```python
from build123d import *

# Parameters (mm, degrees)
F0_W        = 44.3030558527
F0_H        = 33.7232230231
F0_W_2      = 0.2780174837
F0_H_2      = 4.7262893058
F1_DEPTH    = 46.482
F2_T1_DEPTH = 280.6193273788
F3_R        = 21.4623585695
F4_T1_DEPTH = 270.9255150881
F6_DEPTH    = 40.132


# Not quite as in the source:
# - a fillet or chamfer that OpenCascade refuses, or shapes differently, is made with other operations: its cross-section is extruded or revolved along the edge and cut away or added


with BuildPart() as f1:
    # F0 (on Top) → F1 (new body)
    with BuildSketch(Plane.XY):
        with Locations((0.330619514, -6.2817768194)):
            Rectangle(F0_W, F0_H)
        with Locations((8.0964784138, -9.5091590192)):
            Rectangle(F0_W_2, F0_H_2, mode=Mode.SUBTRACT)
    extrude(amount=F1_DEPTH)

    # F2: fillet of radius 49.6700298323 on 1 edges, made by hand

    # F2_s2 → F2_t1 (cut)
    with BuildSketch(Plane.XZ.offset(-134.02788687)):
        with BuildLine():
            ThreePointArc((-21.8209084123, -2.8972208711), (-9.1217429277, 30.2730527625), (22.4821474403, 46.482))
            Line((22.4821474403, 46.482), (-21.8209084123, 46.482))
            Line((-21.8209084123, 46.482), (-21.8209084123, -2.8972208711))
        make_face()
    extrude(amount=F2_T1_DEPTH, mode=Mode.SUBTRACT)

    # F3
    f3_edges = [f1.edges().sort_by_distance(p)[0] for p in [
        (22.482147, -23.143388, 23.241),
    ]]
    fillet(f3_edges, radius=F3_R)

    # F4: fillet of radius 88.3022752574 on 2 edges, made by hand

    # F4_s2 → F4_t1 (cut)
    with BuildSketch(Plane.XY.offset(-112.221757544)):
        with BuildLine():
            ThreePointArc((22.4821474403, -1.6810297614), (0.8599678832, 7.4594865185), (-22.4065555773, 10.5798346922))
            Line((-22.4065555773, 10.5798346922), (22.4821474403, 10.5798346922))
            Line((22.4821474403, 10.5798346922), (22.4821474403, -1.6810297614))
        make_face()
    extrude(amount=F4_T1_DEPTH, mode=Mode.SUBTRACT)

    # F5 (on Front) → F6 (join)
    with BuildSketch(Plane.XZ):
        with BuildLine():
            ThreePointArc((51.0496692561, -13.4370785738), (51.3779423625, -11.1330198173), (51.4876921444, -8.808282204))
            ThreePointArc((51.4876921444, -8.808282204), (50.2324406688, -1.038184698), (46.594391977, 5.9414050633))
            ThreePointArc((46.594391977, 5.9414050633), (46.1598632778, -4.3598915413), (51.0496692561, -13.4370785738))
        make_face()
        with BuildLine():
            ThreePointArc((46.594391977, 5.9414050633), (50.2324406688, -1.038184698), (51.4876921444, -8.808282204))
            ThreePointArc((51.4876921444, -8.808282204), (51.3779423625, -11.1330198173), (51.0496692561, -13.4370785738))
            ThreePointArc((51.0496692561, -13.4370785738), (72.3613537789, -18.0621042721), (84.58179359, 0))
            ThreePointArc((84.58179359, 0), (68.1302794475, 19.2246129703), (46.594391977, 5.9414050633))
        make_face()
        with BuildLine():
            ThreePointArc((51.0496692561, -13.4370785738), (46.1598632778, -4.3598915413), (46.594391977, 5.9414050633))
            ThreePointArc((46.594391977, 5.9414050633), (2.7623791307, -14.3373401751), (51.0496692561, -13.4370785738))
        make_face()
    extrude(amount=-F6_DEPTH)


solid = f1.part
```
Read the model definition and answer for the solid it produces. Units are mm, in the model's axes. Coordinates: 2 decimals unless noted, no trailing zeros. Order: outer loops, then holes, each group sorted by start corner. A loop starts at its lowest first (then second) coordinate and runs counter-clockwise, first axis right, second up. Notation, with made-up numbers: (-15.5, 66.5) - (-1.5, 66.5) arc R14 cw to (-1.5, 92.5) - close; hole circle Ø6 at (23.5, 32.25). An arc over 180 degrees is marked (long way). Answer as a JSON object with one key per item and string values. Group by question number.
Item 1: Section B-B (x = 5.5) is taken. Give the vertices of the cut face in (y, z), plus the area to 3 significant figures.
Item 2: Section A-A (z = 8) is taken. Give the vertices of the cut face in (x, y), plus the area to 3 significant figures.
Item 3: The mould has two halves that part along Y. Classify faces 1 (the face through (8.235, -10, 21)), 2 (the face through (-5, -6, 0)), 3 (the face through (7.957, -10, 21)), 4 (the face through (16.03, -17.02, 23.57)): +Y half, -Y half, draft (parallel to the pull), parting line (faces both ways), or undercut.
Item 4: Section D-D (z = -23) is taken. Give the vertices of the cut face in (x, y), plus the area to 3 significant figures.
Item 5: Section C-C (y = -16) is taken. Give the vertices of the cut face in (x, z).
Item 6: Flat-ended cylindrical pins translate along their axes: P1, Ø2.5, axis at y = -9, z = 18, coming from the +X side; P2, Ø1, axis at x = 12, y = 28, coming from the +Z side; P3, Ø5, axis at x = 42, y = 2, coming from the -Z side. Find the tip coordinate at first contact, or state that the pin passes through.
Item 7: Consider probe 1 along Y at (x, z) = (53.5, 5.5); probe 2 along X at (y, z) = (31.5, 5); probe 3 along Y at (x, z) = (-5.5, 0.5). Determine where each line is inside the solid, lowest interval first. Write a range as from..to.
Results are:
{
 "1": {"outline": "(-22.67, 0) - (0, 0) - (0, -21.25) - (40.13, -21.25) - (40.13, 3.63) - (6.05, 3.63) - (6.05, 41.46) - (-22.67, 41.46) - close", "area": "2,170 mm^2"},
 "2": {"outline": "(-20.61, -23.14) - (1.02, -23.14) arc R21.46 ccw to (22.48, -1.68) arc R88.3 ccw to (19.5, 0) - (44.88, 0) - (44.88, 40.13) - (8.74, 40.13) - (8.74, 4.9) arc R88.3 ccw to (-20.61, 10.56) - close; (47.39, 0) - (82.86, 0) - (82.86, 40.13) - (47.39, 40.13) - close; hole (7.96, -11.87) - (8.24, -11.87) - (8.24, -7.15) - (7.96, -7.15) - close", "area": "4,020 mm^2"},
 "3": {"face 1": "undercut", "face 2": "draft", "face 3": "undercut", "face 4": "-Y half"},
 "4": {"outline": "(6.62, 0) - (47, 0) - (47, 40.13) - (6.62, 40.13) - close", "area": "1,620 mm^2"},
 "5": {"outline": "(-21.74, 0) - (17.01, 0) - (17.01, 45.58) arc R49.67 ccw to start"},
 "6": {"P1": "stops at x = 21.61", "P2": "stops at z = 11.29", "P3": "stops at z = -29.97"},
 "7": {"probe 1": "y = 0..40.13", "probe 2": "x = 6.36..83.93", "probe 3": "y = -23.14..8.95"}
}
